```python
from build123d import *

# Parameters (mm, degrees)
BOSS_EXTRUDE1_DEPTH = 8
SKETCH2_R           = 9.075
CUT_EXTRUDE1_DEPTH  = 4.7
HOLE1_D             = 3.2
HOLE1_CSINK_D       = 6
HOLE1_CSINK_ANGLE   = 90


with BuildPart() as part:
    # Sketch1 → Boss-Extrude1 (new body)
    with BuildSketch(Plane.XY):
        with BuildLine():
            Line((-27.295831523, 0), (-17.704168477, 0))
            ThreePointArc((-17.704168477, 0), (-14.094158417, 2.436015689), (-11.591287885, 6))
            Line((-11.591287885, 6), (-18.346688069, 6))
            ThreePointArc((-18.346688069, 6), (-22.5, 4.5), (-26.653311931, 6))
            Line((-26.653311931, 6), (-33.408712115, 6))
            ThreePointArc((-33.408712115, 6), (-30.905841583, 2.436015689), (-27.295831523, 0))
        make_face()
        with BuildLine():
            Line((-45, 0), (-27.295831523, 0))
            ThreePointArc((-27.295831523, 0), (-30.905841583, 2.436015689), (-33.408712115, 6))
            Line((-33.408712115, 6), (-36, 6))
            Line((-36, 6), (-45, 6))
            Line((-45, 6), (-45, 0))
        make_face()
        with BuildLine():
            Line((-18.346688069, 6), (-11.591287885, 6))
            ThreePointArc((-11.591287885, 6), (-10.82107856, 8.242683552), (-10.506902886, 10.593033646))
            add(Edge.make_bspline(
                [(-10.506902886, 10.593033646), (-10.587978043, 10.993773754), (-10.5, 11)],
                knots=[0.717855618, 0.717855618, 0.717855618, 1, 1, 1], degree=2))
            ThreePointArc((-10.5, 11), (-22.5, 23), (-34.5, 11))
            add(Edge.make_bspline(
                [(-34.493097114, 10.593033646), (-34.412021957, 10.993773754), (-34.5, 11)],
                knots=[0.717855618, 0.717855618, 0.717855618, 1, 1, 1], degree=2))
            ThreePointArc((-34.493097114, 10.593033646), (-34.17892144, 8.242683552), (-33.408712115, 6))
            Line((-33.408712115, 6), (-26.653311931, 6))
            ThreePointArc((-26.653311931, 6), (-25.261654617, 16.884153616), (-16, 11))
            ThreePointArc((-16, 11), (-16.615846384, 8.238345383), (-18.346688069, 6))
        make_face()
        with BuildLine():
            Line((-17.704168477, 0), (0, 0))
            Line((0, 0), (0, 6))
            Line((0, 6), (-9, 6))
            Line((-9, 6), (-11.591287885, 6))
            ThreePointArc((-11.591287885, 6), (-14.094158417, 2.436015689), (-17.704168477, 0))
        make_face()
        with BuildLine():
            ThreePointArc((-34.5, 11), (-34.498274154, 10.796487554), (-34.493097114, 10.593033646))
            add(Edge.make_bspline(
                [(-34.493097114, 10.593033646), (-34.412021957, 10.993773754), (-34.5, 11)],
                knots=[0.717855618, 0.717855618, 0.717855618, 1, 1, 1], degree=2))
        make_face()
        with BuildLine():
            add(Edge.make_bspline(
                [(-10.506902886, 10.593033646), (-10.587978043, 10.993773754), (-10.5, 11)],
                knots=[0.717855618, 0.717855618, 0.717855618, 1, 1, 1], degree=2))
            ThreePointArc((-10.506902886, 10.593033646), (-10.501725846, 10.796487554), (-10.5, 11))
        make_face()
    extrude(amount=BOSS_EXTRUDE1_DEPTH)

    # Sketch2 → Cut-Extrude1 (cut)
    with BuildSketch(Plane.XY.offset(8)):
        with Locations((-22.5, 11)):
            Circle(SKETCH2_R)
    extrude(amount=-CUT_EXTRUDE1_DEPTH, mode=Mode.SUBTRACT)

    # Hole1 (through all)
    with Locations(Plane(origin=(-40, 6, 4), x_dir=(1, 0, 0), z_dir=(0, 1, 0))):
        with Locations((0, 0), (35, 0)):
            CounterSinkHole(HOLE1_D / 2, HOLE1_CSINK_D / 2, counter_sink_angle=HOLE1_CSINK_ANGLE)


solid = part.part
```
Can you work these out from the model? Positions are in its coordinate system, mm. A direction names the side the tool comes from. Coordinates: 2 decimals unless noted, no trailing zeros. Write each loop counter-clockwise with the first axis right and the second up, starting at its lowest first coordinate (ties: lowest second). Pieces come first, ordered by that corner, then holes. Notation, with made-up numbers: M 74,3 L 103,3 A33 cw 103,33 Z; hole C 59,71 d6. An arc over 180 degrees is marked long. Write item = value, one per line. Start each with the question number.
Q1. If we section it at D-D, the plane y = 14.75: Write out the boundary of the cut face in (x, z).
Q2. I'm going to push flat-ended pins straight in: pin 1 (3 mm diameter, centred on x = -15.5, y = 10, fed in from +Z); pin 2 (4 mm diameter, centred on x = -41.5, z = 4, fed in from +Y); pin 3 (1.5 mm diameter, centred on x = -21.5, z = 2, fed in from +Y); pin 4 (11.5 mm diameter, centred on x = -22.5, y = 11, fed in from +Z). Where does each tip first touch, or does it pass through?
Q3. If we section it at C-C, the plane x = -40: Write out the boundary of the cut face in (y, z).
Q4. If we section it at A-A, the plane z = 4: Write out the boundary of the cut face in (x, y) (3 decimals), then the cut area to 3 significant figures.
Q5. Thinking about a two-plate mould opening in Z: for faces 4 (the face through (-3, 5, 4)), 5 (the face through (-8.3, 6, 3.9)), 6 (the face through (-5.86, 2.27, 2.65)), 7 (the face through (-23, 1, 8)), which applies, released by +Z, released by -Z, zero draft, split by the parting line, or undercut?
Q6. If I drill on L1, parallel to Y at x = -22.5, z = 1.9; L2, parallel to Z at x = -40, y = 1.1; L3, parallel to Y at x = -9, z = 0.75, over which ranges is the centre line in solid material (lowest first)? Write a range as [from, to].
Q7. On a 3-axis mill with a long thin cutter (end or side, diameter ignored), from which of +Z, -Z, +X, -X, +Y, -Y can I reach the whole of each face in a straight line? I mean faces 1 (the face through (-36.5, 6, 3.9)), 2 (the face through (-13.844, 13.726, 5.683)), 3 (the face through (-23, 0, 4)). Say none if no direction works.
Q8. If we section it at B-B, the plane z = 0.5: Write out the boundary of the cut face in (x, y), then the cut area to 3 significant figures.
Check sheet entries:
q1.outline = M -33.9,0 L -27.81,0 L -27.81,3.3 L -30.76,3.3 L -30.76,8 L -33.9,8 Z; M -17.19,0 L -11.1,0 L -11.1,8 L -14.24,8 L -14.24,3.3 L -17.19,3.3 Z
q2.pin_1 = 3.3
q2.pin_2 = 6
q2.pin_3 = 23
q2.pin_4 = through
q3.outline = M 0,0 L 6,0 L 6,1 L 4.6,2.4 L 0,2.4 Z; M 0,5.6 L 4.6,5.6 L 6,7 L 6,8 L 0,8 Z
q4.outline = M -45,0 L -41.6,0 L -41.6,4.6 L -43,6 L -45,6 Z; M -38.4,0 L -6.6,0 L -6.6,4.6 L -8,6 L -11.591,6 A12 ccw -10.507,10.593 A12 ccw -10.5,11 A12 ccw -34.5,11 A12 ccw -34.493,10.593 A12 ccw -33.409,6 L -37,6 L -38.4,4.6 Z; M -3.4,0 L 0,0 L 0,6 L -2,6 L -3.4,4.6 Z; hole C -22.5,11 d18.15
q4.area = 312 mm²
q5.face_4 = undercut
q5.face_5 = zero draft
q5.face_6 = undercut
q5.face_7 = released by +Z
q6.L1 = [0, 4.5], [17.5, 23]
q6.L2 = [0, 2.4], [5.6, 8]
q6.L3 = [0, 6]
q7.face_1 = +Z, -Z, -X
q7.face_2 = +Z
q7.face_3 = +Z, -Z, +X, -X, -Y
q8.outline = M -45,0 L 0,0 L 0,6 L -11.59,6 A12 ccw -10.51,10.59 A12 ccw -10.5,11 A12 ccw -34.5,11 A12 ccw -34.49,10.59 A12 ccw -33.41,6 L -45,6 Z; hole C -22.5,11 d13
q8.area = 480 mm²
